The listing builds one solid part. Answer for the finished solid, in the listing's coordinates (mm). A direction names the side the tool comes from. Give positions to 0.01 mm unless a question says otherwise; leave off trailing zeros. Loops run counter-clockwise (first coordinate to the right, second up) from the corner with the lowest first, then second, coordinate; pieces in that order, holes last. Notation, with made-up numbers: M 25,-37.5 L 47,-37.5 A5 ccw 47,-31.5 Z; hole C -37,73 d4. An arc over 180 degrees is marked long. Use one line per item in the form item = value. Start each with the question number.
1. For faces 4 (the face through (35, -25, 5)), 5 (the face through (55, 35, 73)), 6 (the face through (24.853, 2.703, 39.897)), 7 (the face through (101, -25.3, 85)), determine the directions among +Z, -Z, +X, -X, +Y, -Y from which every point of the face is accessible in a straight line to the end or side of a thin tool.
2. Each of these flat-tipped pins is pushed along its axis until it touches: pin 1 Ø5 at (x, y) = (29.5, -3) entering from -Z; pin 2 Ø10 at (y, z) = (28, 61.5) entering from +X; pin 3 Ø1.5 at (x, y) = (-13, -8) entering from +Z. Where does it stop, or does it pass through?
3. The part is cut by section C-C (y = -13). Write down the section's boundary in (x, z).
4. The part is cut by section B-B (z = 14). Write down the section's boundary in (x, y).
5. Straight lines are drawn through the part: line 1 (Y direction, x = 0, z = 38); line 2 (Y direction, x = 0, z = 20); line 3 (Y direction, x = 63, z = 56). For each, find the intervals that lie inside material, in ascending order. Write a range as from..to.
6. The mould has two halves that part along Y. Classify faces 1 (the face through (40, 40, 73)), 2 (the face through (105, 0, 80)), 3 (the face through (45, -2.5, 62)): released by +Y, released by -Y, zero draft, split by the parting line, or undercut.
7. The part is cut by section A-A (y = 0). Write down the section's boundary in (x, z), and give its area (3 significant figures).
8. The part is cut by section D-D (x = 73). Write down the section's boundary in (y, z).
from build123d import *

# Parameters (mm, degrees)
BOSS_EXTRUDE1_DEPTH = 90
CUT_EXTRUDE1_DEPTH  = 10
SKETCH3_R           = 10
CUT_EXTRUDE2_DEPTH  = 166
SKETCH4_R           = 25
CUT_EXTRUDE3_DEPTH  = 50
SKETCH5_R           = 25
CUT_EXTRUDE4_DEPTH  = 10
SKETCH6_R           = 15
CUT_EXTRUDE5_DEPTH  = 148
CUT_EXTRUDE6_DEPTH  = 35
SKETCH8_W           = 10
SKETCH8_H           = 5
CUT_EXTRUDE7_DEPTH  = 145
SKETCH9_W           = 20
SKETCH9_H           = 10
BOSS_EXTRUDE2_DEPTH = 25
CUT_EXTRUDE8_DEPTH  = 10
CUT_EXTRUDE9_DEPTH  = 25
CUT_EXTRUDE10_DEPTH = 25
CUT_EXTRUDE11_DEPTH = 10


with BuildPart() as part:
    # Sketch1 → Boss-Extrude1 (new body)
    with BuildSketch(Plane.XY):
        with BuildLine():
            Line((0, 45), (70, 45))
            ThreePointArc((70, 45), (115, 0), (70, -45))
            Line((70, -45), (0, -45))
            ThreePointArc((0, -45), (-45, 0), (0, 45))
        make_face()
    extrude(amount=BOSS_EXTRUDE1_DEPTH)

    # Sketch2 → Cut-Extrude1 (cut)
    with BuildSketch(Plane(origin=(0, 0, 0), x_dir=(-1, 0, 0), z_dir=(0, 0, -1))):
        with BuildLine():
            Line((0, -25), (-70, -25))
            ThreePointArc((-70, -25), (-95, 0), (-70, 25))
            Line((-70, 25), (0, 25))
            ThreePointArc((0, 25), (25, 0), (0, -25))
        make_face()
    extrude(amount=-CUT_EXTRUDE1_DEPTH, mode=Mode.SUBTRACT)

    # Sketch3 → Cut-Extrude2 (cut)
    with BuildSketch(Plane.XY.offset(90)):
        with Locations((70, 0)):
            Circle(SKETCH3_R)
    extrude(amount=-CUT_EXTRUDE2_DEPTH, mode=Mode.SUBTRACT)

    # Sketch4 → Cut-Extrude3 (cut)
    with BuildSketch(Plane.XY.offset(90)):
        with BuildLine():
            ThreePointArc((12.114503105, -21.868671988), (-25, 0), (12.114503105, 21.868671988))
            Line((12.114503105, 21.868671988), (-20.615528128, 40))
            ThreePointArc((-20.615528128, 40), (-45, 0), (-20.615528128, -40))
            Line((-20.615528128, -40), (12.114503105, -21.868671988))
        make_face()
        Circle(SKETCH4_R)
    extrude(amount=-CUT_EXTRUDE3_DEPTH, mode=Mode.SUBTRACT)

    # Sketch5 → Cut-Extrude4 (cut)
    with BuildSketch(Plane.XY.offset(40)):
        Circle(SKETCH5_R)
    extrude(amount=-CUT_EXTRUDE4_DEPTH, mode=Mode.SUBTRACT)

    # Sketch6 → Cut-Extrude5 (cut)
    with BuildSketch(Plane.XY.offset(30)):
        Circle(SKETCH6_R)
    extrude(amount=-CUT_EXTRUDE5_DEPTH, mode=Mode.SUBTRACT)

    # Sketch7 → Cut-Extrude6 (cut)
    with BuildSketch(Plane.XY.offset(90)):
        with BuildLine():
            Line((40, 45), (0, 45))
            ThreePointArc((0, 45), (-10.606601718, 43.732139211), (-20.615528128, 40))
            Line((-20.615528128, 40), (12.114503105, 21.868671988))
            ThreePointArc((12.114503105, 21.868671988), (25, 0), (12.114503105, -21.868671988))
            Line((12.114503105, -21.868671988), (-20.615528128, -40))
            ThreePointArc((-20.615528128, -40), (-10.606601718, -43.732139211), (0, -45))
            Line((0, -45), (70, -45))
            Line((70, -45), (70, -35))
            ThreePointArc((70, -35), (92.912878475, -26.457513111), (104.641016151, -5))
            Line((104.641016151, -5), (89.641016151, -5))
            ThreePointArc((89.641016151, -5), (49.732550346, 0), (89.641016151, 5))
            Line((89.641016151, 5), (104.641016151, 5))
            ThreePointArc((104.641016151, 5), (92.912878475, 26.457513111), (70, 35))
            Line((70, 35), (40, 35))
            Line((40, 35), (40, 45))
        make_face()
    extrude(amount=-CUT_EXTRUDE6_DEPTH, mode=Mode.SUBTRACT)

    # Sketch8 → Cut-Extrude7 (cut)
    with BuildSketch(Plane(origin=(0, 0, 0), x_dir=(0, 0, -1), z_dir=(1, 0, 0))):
        with Locations((-85, 22.8)):
            Rectangle(SKETCH8_W, SKETCH8_H)
        with Locations((-85, -22.8)):
            Rectangle(SKETCH8_W, SKETCH8_H)
    extrude(amount=CUT_EXTRUDE7_DEPTH, mode=Mode.SUBTRACT)

    # Sketch9 → Boss-Extrude2 (add)
    with BuildSketch(Plane.XY.offset(55)):
        with Locations((40.358983849, 0)):
            Rectangle(SKETCH9_W, SKETCH9_H)
    extrude(amount=BOSS_EXTRUDE2_DEPTH)

    # Sketch10 → Cut-Extrude8 (cut)
    with BuildSketch(Plane.XY.offset(90)):
        with BuildLine():
            Line((89.641016151, 5), (104.641016151, 5))
            ThreePointArc((104.641016151, 5), (102.489767507, 13.015952033), (98.511576596, 20.3))
            Line((98.511576596, 20.3), (110.161050783, 20.3))
            ThreePointArc((110.161050783, 20.3), (115, 0), (110.161050783, -20.3))
            Line((110.161050783, -20.3), (98.511576596, -20.3))
            ThreePointArc((98.511576596, -20.3), (102.489767507, -13.015952033), (104.641016151, -5))
            Line((104.641016151, -5), (89.641016151, -5))
            ThreePointArc((89.641016151, -5), (90.267449654, 0), (89.641016151, 5))
        make_face()
    extrude(amount=-CUT_EXTRUDE8_DEPTH, mode=Mode.SUBTRACT)

    # Sketch11 → Cut-Extrude9 (cut)
    with BuildSketch(Plane.XY.offset(80)):
        with BuildLine():
            Line((49.88732948, -2.5), (30.358983849, -2.5))
            Line((30.358983849, -2.5), (30.358983849, -5))
            Line((30.358983849, -5), (50.358983849, -5))
            ThreePointArc((50.358983849, -5), (50.083890917, -3.757407944), (49.88732948, -2.5))
        make_face()
        with BuildLine():
            Line((50.358983849, 5), (30.358983849, 5))
            Line((30.358983849, 5), (30.358983849, 2.5))
            Line((30.358983849, 2.5), (49.88732948, 2.5))
            ThreePointArc((49.88732948, 2.5), (50.083890917, 3.757407944), (50.358983849, 5))
        make_face()
    extrude(amount=-CUT_EXTRUDE9_DEPTH, mode=Mode.SUBTRACT)

    # Sketch12 → Cut-Extrude10 (cut)
    with BuildSketch(Plane.XY.offset(80)):
        with BuildLine():
            Line((104.910600109, -2.5), (90.11267052, -2.5))
            ThreePointArc((90.11267052, -2.5), (89.916109083, -3.757407944), (89.641016151, -5))
            Line((89.641016151, -5), (104.641016151, -5))
            ThreePointArc((104.641016151, -5), (104.798266209, -3.752421735), (104.910600109, -2.5))
        make_face()
        with BuildLine():
            Line((104.641016151, 5), (89.641016151, 5))
            ThreePointArc((89.641016151, 5), (89.916109083, 3.757407944), (90.11267052, 2.5))
            Line((90.11267052, 2.5), (104.910600109, 2.5))
            ThreePointArc((104.910600109, 2.5), (104.798266209, 3.752421735), (104.641016151, 5))
        make_face()
    extrude(amount=-CUT_EXTRUDE10_DEPTH, mode=Mode.SUBTRACT)

    # Sketch13 → Cut-Extrude11 (cut)
    with BuildSketch(Plane.XZ.offset(2.5)):
        Polygon((49.88732948, 80), (30.358983849, 55), (30.358983849, 80), align=None)
    extrude(amount=-CUT_EXTRUDE11_DEPTH, mode=Mode.SUBTRACT)


solid = part.part
Derived:
q1.face_4 = -Z
q1.face_5 = +Z, -X
q1.face_6 = +Z
q1.face_7 = +Z, +X, -X
q2.pin_1 = 10
q2.pin_2 = 108.68
q2.pin_3 = 30
q3.outline = M -43.08,0 L -21.35,0 L -21.35,10 L -7.48,10 L -7.48,30 L -21.35,30 L -21.35,40 L -43.08,40 Z; M 7.48,10 L 91.35,10 L 91.35,0 L 113.08,0 L 113.08,80 L 102.5,80 L 102.5,55 L 85.55,55 L 85.55,90 L 54.45,90 L 54.45,55 L 21.35,55 L 21.35,30 L 7.48,30 Z
q4.outline = M 0,-45 L 70,-45 A45 ccw 70,45 L 0,45 A45 ccw Z; hole C 0,0 d30; hole C 70,0 d20
q5.line_1 = -45..-25, 25..45
q5.line_2 = -45..-15, 15..45
q5.line_3 = -19.02..-7.14, 7.14..19.02, 35..45
q6.face_1 = zero draft
q6.face_2 = undercut
q6.face_3 = released by -Y
q7.outline = M -45,0 L -25,0 L -25,10 L -15,10 L -15,30 L -25,30 L -25,40 L -45,40 Z; M 15,10 L 60,10 L 60,90 L 49.73,90 L 49.73,80 L 49.89,80 L 30.36,55 L 25,55 L 25,30 L 15,30 Z; M 80,10 L 95,10 L 95,0 L 115,0 L 115,80 L 90.27,80 L 90.27,90 L 80,90 Z
q7.area = 6,130 mm2
q8.outline = M -44.9,0 L -24.82,0 L -24.82,10 L -9.54,10 L -9.54,90 L -20.04,90 L -20.04,55 L -34.87,55 L -34.87,90 L -44.9,90 Z; M 9.54,10 L 24.82,10 L 24.82,0 L 44.9,0 L 44.9,90 L 34.87,90 L 34.87,55 L 20.04,55 L 20.04,90 L 9.54,90 Z
